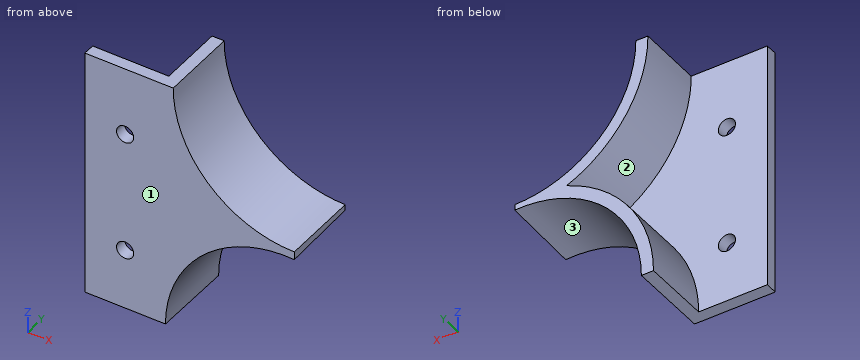
from build123d import *

# Parameters (mm, degrees)
SKETCH_1_W               = 50
SKETCH_1_H               = 60
EXTRUDE_1_DEPTH          = 70
DRAFT_1_ANGLE            = 1.591
CUT_EXTRUDE_1_DEPTH      = 72
CUT_EXTRUDE_1_DEPTH_BACK = 2
SKETCH_3_R               = 30
SKETCH_4_R               = 30
CUT_EXTRUDE_2_DEPTH      = 70
SKETCH_5_W               = 61.388766385
SKETCH_5_H               = 50
CUT_EXTRUDE_3_DEPTH      = 93.836652759
SHELL_1_T                = -3
SKETCH_6_R               = 2.125
CUT_EXTRUDE_4_DEPTH      = 64.305956024


with BuildPart() as part:
    # 草圖1 → 填料-伸長1 (new body)
    with BuildSketch(Plane(origin=(0, 0, 0), x_dir=(1, 0, 0), z_dir=(0, 1, 0))):
        with Locations((25, 0)):
            Rectangle(SKETCH_1_W, SKETCH_1_H)
    extrude(amount=EXTRUDE_1_DEPTH)

    # 拔模1
    draft_1_faces = [part.faces().sort_by_distance(p)[0] for p in [
        (50, 35, 0),
        (25, 35, 30),
    ]]
    draft(draft_1_faces, Plane.ZX.offset(70), DRAFT_1_ANGLE)

    # 草圖3 → 除料-伸長1 (cut, two sides: drawn at the far end of the back side and taken through both)
    with BuildSketch(Plane(origin=(50, 70, 30), x_dir=(0.9996147856379402, 0.02774322520612563, -0.0007705771714084017), z_dir=(0.02775392465967472, -0.9992294227713525, 0.027753924659674706)).offset(-CUT_EXTRUDE_1_DEPTH_BACK)):
        Circle(SKETCH_3_R)
    extrude(amount=CUT_EXTRUDE_1_DEPTH + CUT_EXTRUDE_1_DEPTH_BACK, mode=Mode.SUBTRACT)

    # 草圖4 → 除料-伸長2 (cut)
    with BuildSketch(Plane(origin=(0, 70, 0), x_dir=(1, 0, 0), z_dir=(0, 1, 0))):
        with Locations((50, 30)):
            Circle(SKETCH_4_R)
    extrude(amount=-CUT_EXTRUDE_2_DEPTH, mode=Mode.SUBTRACT)

    # 草圖5 → 除料-伸長3 (cut, through all)
    with BuildSketch(Plane.ZY):
        with Locations((0.694383192, 45)):
            Rectangle(SKETCH_5_W, SKETCH_5_H)
    extrude(amount=-CUT_EXTRUDE_3_DEPTH, mode=Mode.SUBTRACT)

    # 薄殼1
    shell_1_openings = [part.faces().sort_by_distance(p)[0] for p in [
        (14.866961876, 20, 1.073459526),
        (10, 10, -30),
        (10.828073147, 9.957245624, 31.667707178),
        (0, 9.984986274, 0.833468336),
    ]]
    offset(amount=SHELL_1_T, openings=shell_1_openings, kind=Kind.INTERSECTION)

    # 草圖6 → 除料-伸長4 (cut, through all)
    with BuildSketch(Plane(origin=(0, 3, 0), x_dir=(1, 0, 0), z_dir=(0, 1, 0))):
        with Locations(Location((10, 15, 0), (0, 0, 270))):
            Circle(SKETCH_6_R)
        with Locations(Location((10, -15, 0), (0, 0, 90))):
            Circle(SKETCH_6_R)
    extrude(amount=-CUT_EXTRUDE_4_DEPTH, mode=Mode.SUBTRACT)


solid = part.part
Read the model definition and answer for the solid it produces. Units are mm, in the model's axes. Face numbers are marked on the shaded views. Give positions to 0.01 mm unless a question says otherwise; leave off trailing zeros. Write each loop counter-clockwise with the first axis right and the second up, starting at its lowest first coordinate (ties: lowest second). Pieces come first, ordered by that corner, then holes. Notation, with made-up numbers: M 71.25,17 L 101.25,17 A8 ccw 101.25,29 Z; hole C -7.5,15 d6. An arc over 180 degrees is marked long. One line per item, written item: value. Start each with the question number.
(1) Determine the mould class of the marked faces 1, 2 and 3 for opening direction Z: pulls with the +Z half, pulls with the -Z half, needs draft (parallel to the pull), parting line crosses it, or undercut.
(2) Find section C-C (z = -8). Determine the outline of the cut face in (x, y), plus the area to 3 significant figures.
(3) Find section B-B (z = -15). Determine the outline of the cut face in (x, y) (3 decimals), plus the area to 3 significant figures.
(4) Find the intervals of material crossed by line 1 (Z direction, x = 24, y = 5); line 2 (Y direction, x = 16, z = -23); line 3 (X direction, y = 1.45, z = -15) (3 decimals), in increasing order.
(5) Flat-ended cylindrical pins translate along their axes: pin 1 Ø6 at (y, z) = (16, -6) entering from +X; pin 2 Ø8 at (x, z) = (11, -14) entering from +Y; pin 3 Ø1 at (x, y) = (42, 15.5) entering from +Z. Find the tip coordinate at first contact, or state that the pin passes through.
(6) Find section A-A (x = 10). Determine the outline of the cut face in (y, z) (3 decimals), plus the area to 3 significant figures.
Results below:
1. face 1: needs draft
1. face 2: undercut
1. face 3: pulls with the -Z half
2. outline: M 0,0 L 29.6,0 L 29.6,20 L 25.4,20 L 25.4,3 L 0,3 Z
2. area: 160 mm^2
3. outline: M 0,0 L 7.875,0 L 7.875,3 L 0,3 Z; M 12.125,0 L 24.019,0 L 24.019,20 L 20.606,20 L 20.606,3 L 12.125,3 Z
3. area: 117 mm^2
4. line 1: z = -15.03 to -9.68, 13.99 to 20.49
4. line 2: y = 0 to 3
4. line 3: x = 0 to 7.875, 12.125 to 24.019
5. pin 1: stops at x = 36.92
5. pin 2: stops at y = 3
5. pin 3: stops at z = 3.22
6. outline: M 0,-30 L 3,-30 L 3,-17.125 L 0,-17.125 Z; M 0,-12.875 L 3,-12.875 L 3,12.875 L 0,12.875 Z; M 0,17.125 L 3,17.125 L 3,31.861 L 0,31.944 Z
6. area: 160 mm^2
